Could you check a few things on this model? Use its own coordinates, in mm. Give positions to 0.01 mm unless a question says otherwise; leave off trailing zeros. Order: outer loops, then holes, each group sorted by start corner. A loop starts at its lowest first (then second) coordinate and runs counter-clockwise, first axis right, second up. Notation, with made-up numbers: (84, 83) - (139, 83) arc R19 cw to (139, 92) - close; hole circle Ø7 at (88, 58). An arc over 180 degrees is marked (long way). Put each result on its own line as item: value.
Autodesk Inventor part; units mm, degrees
ref_plane "YZ Plane" through (0, 0, 0) normal (1, 0, 0) x (0, 1, 0)
ref_plane "XZ Plane" through (0, 0, 0) normal (0, 1, 0) x (-1, 0, 0)
ref_plane "XY Plane" through (0, 0, 0) normal (0, 0, 1) x (1, 0, 0)
sketch "Skizze1" plane through (0, 0, 0) normal (0, 1, 0) x (-1, 0, 0)
  circle A0 centre (0, 0) radius 1.5
  dimension "d0" = 3
extrude "Extrusion1" add sketch "Skizze1" along normal blind 4
sketch "Skizze2" plane through (0, 4, 0) normal (0, 1, 0) x (1, 0, 0)
  circle A0 centre (0, 0) radius 1
  dimension "d3" = 2
extrude "Extrusion2" add sketch "Skizze2" along normal blind 3
sketch "Skizze3" plane through (0, 0, 0) normal (0, 0, 1) x (1, 0, 0)
  circle A0 centre (0, 2.1465) radius 1
  point P0 (0, 0)
  dimension "d6" = 2
extrude "Extrusion3" cut sketch "Skizze3" along normal mid plane 6
properties part number "P_Servo_SIMPROP_ex"
1) Suppose I cut it at D-D, the plane y = 3. List the corners of the cut face in (x, z) for me.
Filled in:
outline: (-0.52, -1.41) - (-0.52, 1.41) arc R1.5 ccw to start; (0.52, -1.41) arc R1.5 ccw to (0.52, 1.41) - close
2) Suppose I cut it at A-A, the plane x = 0. List the corners of the cut face in (y, z) for me.
Filled in:
outline: (0, -1.5) - (1.15, -1.5) - (1.15, 1.5) - (0, 1.5) - close; (3.15, -1.5) - (4, -1.5) - (4, -1) - (7, -1) - (7, 1) - (4, 1) - (4, 1.5) - (3.15, 1.5) - close
3) Suppose I cut it at C-C, the plane z = -1.25. List the corners of the cut face in (x, y) for me.
Filled in:
outline: (-0.83, 0) - (0.83, 0) - (0.83, 1.59) arc R1 cw to (-0.83, 1.59) - close; (-0.83, 2.71) arc R1 cw to (0.83, 2.71) - (0.83, 4) - (-0.83, 4) - close
4) Suppose I cut it at B-B, the plane z = -0.15. List the corners of the cut face in (x, y) for me, and give its area (3 significant figures).
Filled in:
outline: (-1.49, 0) - (1.49, 0) - (1.49, 4) - (0.99, 4) - (0.99, 7) - (-0.99, 7) - (-0.99, 4) - (-1.49, 4) - close; hole circle Ø2 at (0, 2.15)
area: 14.7 mm^2
5) We'd pull the mould along Y, two halves only. Please class faces 1 (the cylindrical face through (0, 5, -1)), 2 (the flat face through (0, 7, 0)), 3 (the cylindrical face through (0.954, 1.846, -0.021)), 4 (the flat face through (0, 0, 0)): pulls with the +Y half, pulls with the -Y half, needs draft (parallel to the pull), parting line crosses it, or undercut.
Filled in:
face 1: needs draft
face 2: pulls with the +Y half
face 3: undercut
face 4: pulls with the -Y half
6) I'm going to push flat-ended pins straight in: pin 1 (1 mm diameter, centred on y = 2, z = 0.5, fed in from -X); pin 2 (1.5 mm diameter, centred on x = -0.5, y = 5, fed in from -Z). Where does each tip first touch, or does it pass through?
Filled in:
pin 1: stops at x = -1.5
pin 2: stops at z = -1
7) If I drill on line 1 (Y direction, x = 0, z = -0.5); line 2 (X direction, y = 1.75, z = -1); line 3 (X direction, y = 3, z = 0.7), over which ranges is the centre line in solid material (lowest first)? Write a range as [from, to].
Filled in:
line 1: y = [0, 1.15], [3.15, 7]
line 2: x = [-1.12, -0.92], [0.92, 1.12]
line 3: x = [-1.33, -0.52], [0.52, 1.33]
